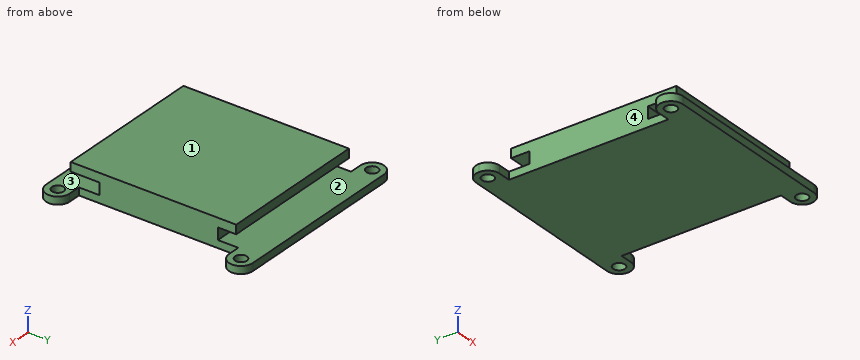
from build123d import *

# Parameters (mm, degrees)
SKETCH073_W  = 32
SKETCH073_H  = 44
PAD037_DEPTH = 1.6
SKETCH074_W  = 32
SKETCH074_H  = 25.2
PAD038_DEPTH = 2.5
SKETCH075_W  = 32
SKETCH075_H  = 35.2
PAD039_DEPTH = 1.9
SKETCH076_R  = 1.25
PAD040_DEPTH = 1.6


with BuildPart() as part:
    # Sketch073 → Pad037 (new body)
    with BuildSketch(Plane.XY):
        Rectangle(SKETCH073_W, SKETCH073_H)
    extrude(amount=PAD037_DEPTH)

    # Sketch074 → Pad038 (join)
    with BuildSketch(Plane.XY.offset(1.6)):
        Rectangle(SKETCH074_W, SKETCH074_H)
    extrude(amount=PAD038_DEPTH)

    # Sketch075 → Pad039 (join)
    with BuildSketch(Plane.XY.offset(4.1)):
        with Locations((0, -1.1)):
            Rectangle(SKETCH075_W, SKETCH075_H)
    extrude(amount=PAD039_DEPTH)

    # Sketch076 → Pad040 (join)
    with BuildSketch(Plane.XY):
        with BuildLine():
            Line((16, 22), (16, 16.95))
            Line((16, 16.95), (18.625, 16.95))
            ThreePointArc((18.625, 16.95), (21.15, 19.475), (18.625, 22))
            Line((18.625, 22), (16, 22))
        make_face()
        with Locations((18.625, 19.475)):
            Circle(SKETCH076_R, mode=Mode.SUBTRACT)
        with BuildLine():
            Line((16, -22), (18.625, -22))
            ThreePointArc((18.625, -22), (21.15, -19.475), (18.625, -16.95))
            Line((18.625, -16.95), (16, -16.95))
            Line((16, -16.95), (16, -22))
        make_face()
        with Locations((18.625, -19.475)):
            Circle(SKETCH076_R, mode=Mode.SUBTRACT)
        with BuildLine():
            Line((-16, -22), (-16, -16.95))
            Line((-16, -16.95), (-18.625, -16.95))
            ThreePointArc((-18.625, -16.95), (-21.15, -19.475), (-18.625, -22))
            Line((-18.625, -22), (-16, -22))
        make_face()
        with Locations((-18.625, -19.475)):
            Circle(SKETCH076_R, mode=Mode.SUBTRACT)
        with BuildLine():
            Line((-16, 22), (-18.625, 22))
            ThreePointArc((-18.625, 22), (-20.410445, 21.260445), (-21.15, 19.475))
            ThreePointArc((-21.15, 19.475), (-20.410445, 17.689555), (-18.625, 16.95))
            Line((-18.625, 16.95), (-16, 16.95))
            Line((-16, 16.95), (-16, 22))
        make_face()
        with Locations((-18.625, 19.475)):
            Circle(SKETCH076_R, mode=Mode.SUBTRACT)
    extrude(amount=PAD040_DEPTH)


with BuildPart() as part_1:
    # Body011 placement: moved
    add(part.part.moved(Location((0, 12, 19.1))))


solid = part_1.part
Could you check a few things on this model? Use its own coordinates, in mm. Face numbers are marked on the shaded views. A direction names the side the tool comes from. Give positions to 0.01 mm unless a question says otherwise; leave off trailing zeros. Order: outer loops, then holes, each group sorted by start corner. A loop starts at its lowest first (then second) coordinate and runs counter-clockwise, first axis right, second up.
1. Suppose I cut it at A-A (y = -3). List the corners of the cut face in (x, z) for me.
2. We'd pull the mould along Y, two halves only. Please class the marked faces 3 and 4: pulls with the +Y half, pulls with the -Y half, needs draft (parallel to the pull), parting line crosses it, or undercut.
3. For the marked faces 1 and 2, which set-ups out of +Z, -Z, +X, -X, +Y, -Y let a thin tool reach every point of the face, with its end or its side?
4. Will these pins go through, and if not, where does the flat tip stop? P1, Ø3, axis at y = 15, z = 21.5, coming from the -X side; P2, Ø4, axis at x = -18.625, y = 31.475, coming from the +Z side; P3, Ø1.2, axis at x = 4, z = 21.5, coming from the -Y side; P4, Ø3, axis at x = 18.625, y = -7.475, coming from the -Z side.
5. I need wall thicknesses on L1, parallel to X at y = -7, z = 20.2; L2, parallel to Z at x = 5.5, y = -2.5; L3, parallel to X at y = 19.5, z = 22.9. Which ranges of each line are inside material? Lowest first, please.
6. Suppose I cut it at C-C (x = -18). List the corners of the cut face in (y, z) for me.
7. Suppose I cut it at D-D (z = 24.5). List the corners of the cut face in (x, y) for me.
8. Suppose I cut it at B-B (x = -5). List the corners of the cut face in (y, z) for me.
Solved:
1. outline: (-16, 19.1) - (16, 19.1) - (16, 20.7) - (-16, 20.7) - close; (-16, 23.2) - (16, 23.2) - (16, 25.1) - (-16, 25.1) - close
2. face 3: needs draft
2. face 4: undercut
3. face 1: +Z, +X, -X, +Y, -Y
3. face 2: +X, -X, +Y
4. P1: stops at x = -16
4. P2: stops at z = 20.7
4. P3: stops at y = -0.6
4. P4: stops at z = 19.1
5. L1: x = -21.1 to -19.78, -17.47 to 17.47, 19.78 to 21.1
5. L2: z = 19.1 to 20.7, 23.2 to 25.1
5. L3: x = -16 to 16
6. outline: (-10, 19.1) - (-8.56, 19.1) - (-8.56, 20.7) - (-10, 20.7) - close; (-6.39, 19.1) - (-4.95, 19.1) - (-4.95, 20.7) - (-6.39, 20.7) - close; (28.95, 19.1) - (30.39, 19.1) - (30.39, 20.7) - (28.95, 20.7) - close; (32.56, 19.1) - (34, 19.1) - (34, 20.7) - (32.56, 20.7) - close
7. outline: (-16, -6.7) - (16, -6.7) - (16, 28.5) - (-16, 28.5) - close
8. outline: (-10, 19.1) - (34, 19.1) - (34, 20.7) - (24.6, 20.7) - (24.6, 23.2) - (28.5, 23.2) - (28.5, 25.1) - (-6.7, 25.1) - (-6.7, 23.2) - (-0.6, 23.2) - (-0.6, 20.7) - (-10, 20.7) - close
